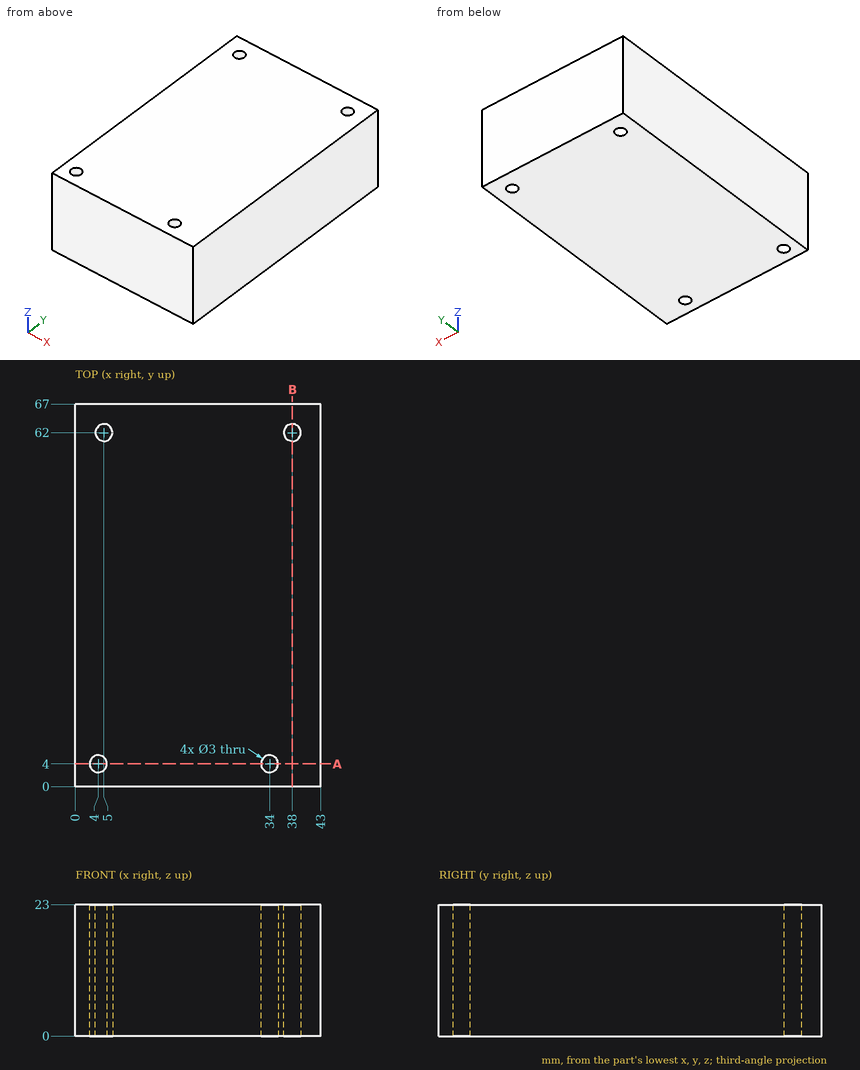
Verification items for this drawing (mm, ordinates from the low corner). Round coordinates to 2 decimals unless told otherwise and drop trailing zeros. Loops run counter-clockwise (first coordinate to the right, second up) from the corner with the lowest first, then second, coordinate; pieces in that order, holes last. Notation, with made-up numbers: (-23, 30.25) -> (31, 30.25) arc R22 ccw to (31, 50.25) -> close; hole circle Ø3 at (27, 25). An arc over 180 degrees is marked (long way). Write item = value, one per line. Start each with the question number.
1) Sectioned sample at A-A, the plane y = 4. Record the cut outline in (x, z).
2) Sectioned sample at B-B, the plane x = 38. Record the cut outline in (y, z).
3) Thickness scan on probe 1 along Y at (x, z) = (5, 13.5); probe 2 along Y at (x, z) = (34, 6.5); probe 3 along Y at (x, z) = (4, 9.25). Record the ranges inside material, lowest first.
4) Gauge pin test, flat end, axial feed: pin 1 Ø2.5 at (x, y) = (34, 4) entering from +Z. Record the tip position at first contact, or that the pin passes through.
Results are:
q1.outline = (0, 0) -> (2.5, 0) -> (2.5, 23) -> (0, 23) -> close; (5.5, 0) -> (32.5, 0) -> (32.5, 23) -> (5.5, 23) -> close; (35.5, 0) -> (43, 0) -> (43, 23) -> (35.5, 23) -> close
q2.outline = (0, 0) -> (60.5, 0) -> (60.5, 23) -> (0, 23) -> close; (63.5, 0) -> (67, 0) -> (67, 23) -> (63.5, 23) -> close
q3.probe_1 = 0 to 2.88, 5.12 to 60.5, 63.5 to 67
q3.probe_2 = 0 to 2.5, 5.5 to 67
q3.probe_3 = 0 to 2.5, 5.5 to 60.88, 63.12 to 67
q4.pin_1 = through
